from build123d import *

# Parameters (mm, degrees)
F0_W      = 26.15
F0_H      = 11
F1_DEPTH  = 16.15
F3_DEPTH  = 25
F5_DEPTH  = 1
F13_DEPTH = 10


# Not quite as in the source:
# - the program builds the solid bodies; features that only make, move or delete a surface that nothing else refers to are left out


with BuildPart() as f1:
    # F0 (on Right) → F1 (new body)
    with BuildSketch(Plane.YZ):
        with Locations((6.6714687273, -5.5)):
            Rectangle(F0_W, F0_H)
    extrude(amount=F1_DEPTH)

    # F2 (on face) → F3 (cut)
    with BuildSketch(Plane(origin=(0, 0, 0), x_dir=(0, -1, 0), z_dir=(-1, 0, 0))):
        Polygon((-19.7464687273, -6.7590326071), (6.4035312727, 0), (-19.7464687273, 0), align=None)
    extrude(amount=-F3_DEPTH, mode=Mode.SUBTRACT)

    # F4 (on face) → F5 (cut)
    with BuildSketch(Plane(origin=(0, -0.4010136369, -1.5514803987), x_dir=(1, 0, 0), z_dir=(0, 0.2502475322, 0.9681818903))):
        with BuildLine():
            Line((12.7111524343, 0), (12.7111524343, 20.8096046483))
            Line((12.7111524343, 20.8096046483), (8.075, 20.8096046483))
            Line((8.075, 20.8096046483), (8.075, -2.8755263988))
            ThreePointArc((8.075, -2.8755263988), (11.1931797197, -2.7277537217), (12.7111524343, 0))
        make_face()
    extrude(amount=-F5_DEPTH, mode=Mode.SUBTRACT)

    # F9 (on offset) → F10 (revolve, cut)
    with BuildSketch(Plane.YZ.offset(6)):
        Polygon((7.6412414201, -3.6817420176), (-6.7182444036, -3.1987416248), (-6.7182444036, -6.9507951848), (7.6412414201, -6.9507951848), align=None)
        Polygon((19.8289547116, -6.5558860078), (7.6412414201, -3.6817420176), (7.6412414201, -6.9507951848), (19.8289547116, -6.9507951848), align=None)
    revolve(axis=Axis((6, 0.4614985082, -6.9507951848), (0, -1, 0)), mode=Mode.SUBTRACT)

    # F9 (on offset) → F11 (revolve, cut)
    with BuildSketch(Plane.YZ.offset(6)):
        Polygon((19.8289547116, -6.5558860078), (7.6412414201, -3.6817420176), (7.6412414201, -6.9507951848), (19.8289547116, -6.9507951848), align=None)
    revolve(axis=Axis((6, 13.7350980658, -6.9507951848), (0, 1, 0)), mode=Mode.SUBTRACT)

    # F12 (on face) → F13 (cut)
    with BuildSketch(Plane(origin=(0, -0.4010136369, -1.5514803987), x_dir=(1, 0, 0), z_dir=(0, 0.2502475322, 0.9681818903))):
        with BuildLine():
            Line((0, 13.5377381568), (0, 2.3293004092))
            ThreePointArc((0, 2.3293004092), (1.4062806348, 7.933519283), (0, 13.5377381568))
        make_face()
        with BuildLine():
            Line((16.15, 2.3293004092), (16.15, 13.5377381568))
            ThreePointArc((16.15, 13.5377381568), (14.7437193652, 7.933519283), (16.15, 2.3293004092))
        make_face()
    extrude(amount=-F13_DEPTH, mode=Mode.SUBTRACT)


solid = f1.part
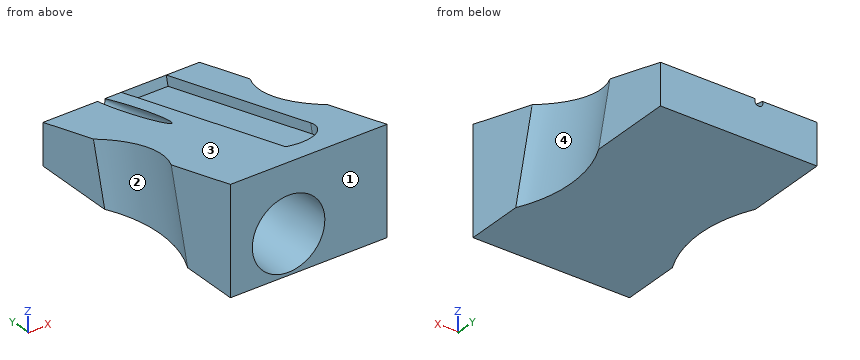
Geometry: final body of the model. Coordinates: model frame, mm. Face numbers are marked on the shaded views. Coordinates: 2 decimals unless noted, no trailing zeros. Loops run counter-clockwise (first coordinate to the right, second up) from the corner with the lowest first, then second, coordinate; pieces in that order, holes last. Notation, with made-up numbers: (80, 27) - (104, 27) arc R30 ccw to (104, 52) - close; hole circle Ø7 at (28.5, 38). An arc over 180 degrees is marked (long way). Put each result on its own line as item: value. Start each with the question number.
Q1. Cut plane A-A, the plane y = 15.5. Return loops of the section in (x, z) (3 decimals).
Q2. Cut plane B-B, the plane x = 6. Return loops of the section in (y, z).
Q3. Pull-direction query (Y, two-part tool) for the marked faces 1, 2, 3 and 4; classes: released by +Y, released by -Y, zero draft, split by the parting line, or undercut.
Q4. Line query: line 1 (X direction, y = 15.5, z = -6) (3 decimals); line 2 (Z direction, x = 6.75, y = 0.5); line 3 (X direction, y = -0.25, z = -2.5) (3 decimals). Output: solid intervals per line, ascending.
Q5. Cut plane C-C, the plane x = 14. Return loops of the section in (y, z).
Q6. Pin query (flat end, axial travel): pin 1 Ø3.5 at (y, z) = (9, -3.5) entering from +X; pin 2 Ø3 at (y, z) = (13, -3) entering from +X; pin 3 Ø3 at (y, z) = (10.5, -5) entering from -X; pin 4 Ø1.5 at (x, y) = (13.5, 2) entering from +Z. Return the tip coordinate at first contact, or that it passes through.
Q7. Cut plane D-D, the plane x = 10.25. Return loops of the section in (y, z), and give its area (3 significant figures).
Filled sheet:
1. outline: (0, -11) - (16.15, -11) - (16.15, -5.661) - (12.711, -5.661) - (12.711, -6.694) - (8.075, -6.694) - (8.075, -5.661) - (6.585, -5.661) arc R1.416 cw (long way) to (5.415, -5.661) - (0, -5.661) - close
2. outline: (-6.4, -11) - (19.75, -11) - (19.75, -7.37) - (7.64, -10.22) - (-6.4, -10.69) - close; (-6.4, -3.21) - (7.64, -3.68) - (9.92, -4.22) - (-6.4, 0) - close
3. face 1: released by -Y
3. face 2: undercut
3. face 3: released by +Y
3. face 4: undercut
4. line 1: 0 to 4.951, 7.049 to 8.075, 12.711 to 16.15
4. line 2: -11 to -10.38, -3.52 to -1.78
4. line 3: 0 to 8.075, 12.711 to 16.15
5. outline: (-6.4, -11) - (19.75, -11) - (19.75, -6.76) - (-6.4, 0) - close
6. pin 1: x = 15.22
6. pin 2: through
6. pin 3: x = 0.31
6. pin 4: z = -1.98
7. outline: (-6.4, -11) - (19.75, -11) - (19.75, -6.76) - (19.5, -7.73) - (-3.67, -1.74) - (-3.42, -0.77) - (-6.4, 0) - close
7. area: 175 mm²
